Geometry: see drawing. Coordinates: mm, zero at the bounding-box minimum. Give positions to 0.01 mm unless a question says otherwise; leave off trailing zeros. Write each loop counter-clockwise with the first axis right and the second up, starting at its lowest first coordinate (ties: lowest second). Pieces come first, ordered by that corner, then holes. Notation, with made-up numbers: (-19.75, 37) -> (33.25, 37) arc R17 ccw to (33.25, 46) -> close; hole circle Ø6 at (24.5, 37.5). An arc over 180 degrees is marked (long way). Answer as a JSON object with one key per item and string values. Group by question number.
Item 1: Section query A-A on x = 33. Return the cut outline in (y, z) (1 decimal).
Item 2: Section query D-D on z = 179. Return the cut outline in (x, y) (1 decimal).
Item 3: Section query C-C on z = 68. Return the cut outline in (x, y), plus the area to 3 significant figures.
Item 4: First-contact query: pin 1 Ø6 at (y, z) = (58.5, 29.5) entering from -X; pin 2 Ø8 at (x, z) = (13, 165.5) entering from +Y; pin 3 Ø2 at (y, z) = (48.5, 36) entering from -X. Flat tips, straight axial feed; report the tip coordinate or a pass-through.
Item 5: Ray query, probe 1 along Y at (x, z) = (34, 50.5) (1 decimal); probe 2 along Z at (x, y) = (47.5, 35.5) (1 decimal); probe 3 along Z at (x, y) = (52.5, 29). Return the intervals inside material, ascending. Write a range as from..to.
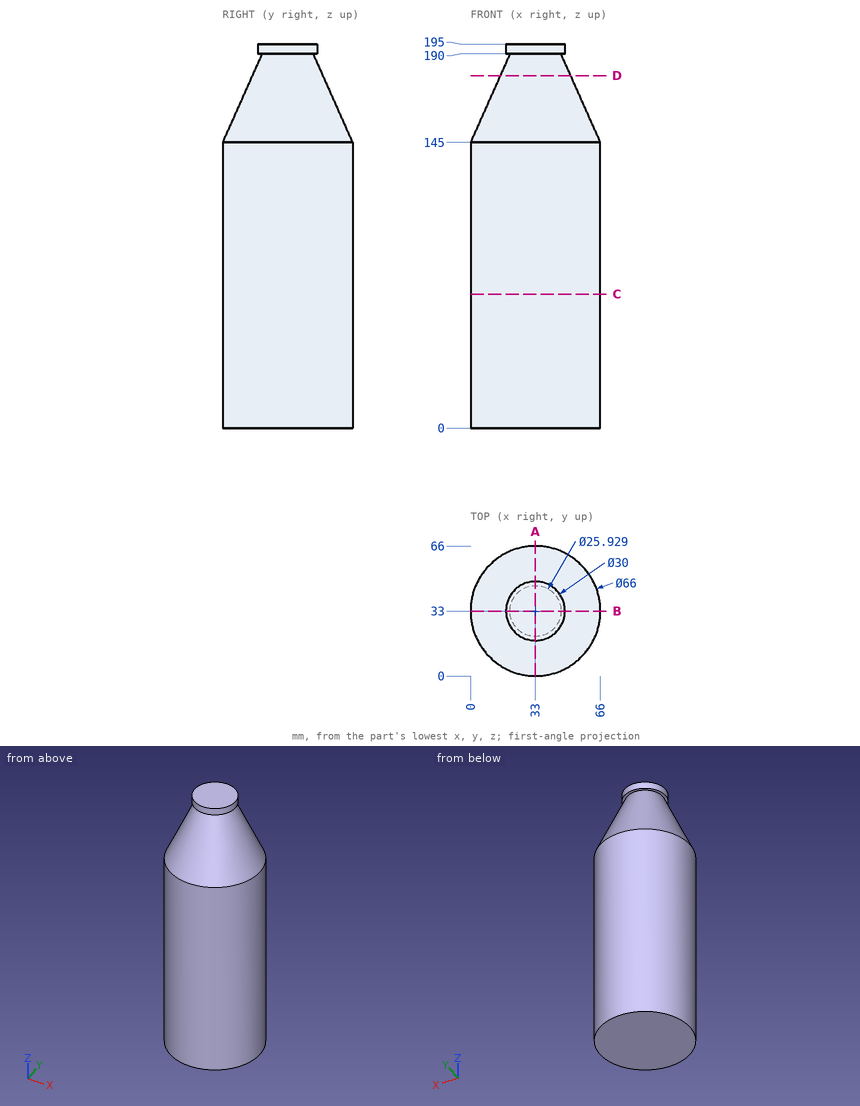
Worked answers:
{
 "1": {"outline": "(0, 0) -> (66, 0) -> (66, 145) -> (46, 190) -> (48, 190) -> (48, 195) -> (18, 195) -> (18, 190) -> (20, 190) -> (0, 145) -> close"},
 "2": {"outline": "circle Ø35.7 at (33, 33)"},
 "3": {"outline": "circle Ø66 at (33, 33)", "area": "3,420 mm^2"},
 "4": {"pin 1": "x = 8.86", "pin 2": "y = 51.44", "pin 3": "x = 3.36"},
 "5": {"probe 1": "0..66", "probe 2": "0..186.1, 190..195", "probe 3": "0..174.41"}
}
